Could you check a few things on this model? Use its own coordinates, in mm. Face numbers are marked on the shaded views. A direction names the side the tool comes from. Round coordinates to 2 decimals unless told otherwise and drop trailing zeros. Loops run counter-clockwise (first coordinate to the right, second up) from the corner with the lowest first, then second, coordinate; pieces in that order, holes last. Notation, with made-up numbers: (-21.75, -7) -> (31.25, -7) arc R30 ccw to (31.25, 32) -> close; hole circle Ø2 at (48.5, -31.5). An arc over 180 degrees is marked (long way). Write each question's results on one line, items separated by ' | '. Start each with the question number.
1) If I drill on probe 1 along Z at (x, y) = (-0.75, 39); probe 2 along Z at (x, y) = (-3.25, 6), over which ranges is the centre line in solid material (lowest first)?
2) Imagine slicing it at B-B, the plane x = -3.75. List the corners of the cut face in (y, z) for me.
3) Imagine slicing it at A-A, the plane y = 53.5. List the corners of the cut face in (x, z) for me.
4) For P1, Ø3, axis at y = 59, z = -4, coming from the -X side; P2, Ø2, axis at y = 58, z = -4, coming from the +X side, each with a flat end and sliding along its axis, tell me the tip position at first contact or that it passes through.
5) Which directions (+Z, -Z, +X, -X, +Y, -Y) give clear straight access to the entire face, cutting with the end or side of a thin tool? Please do the marked faces 1, 2 and 3.
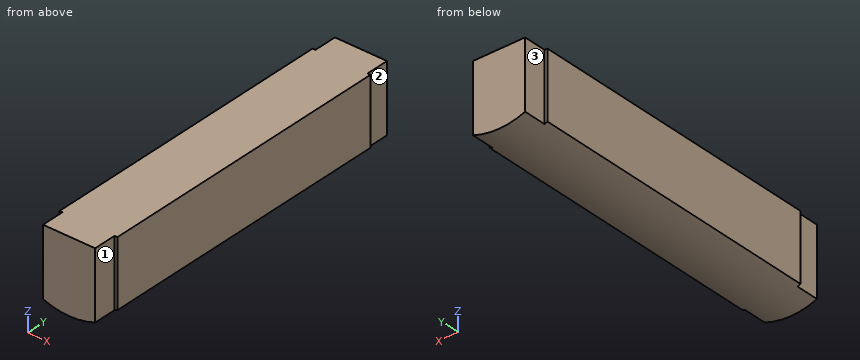
from build123d import *

# Parameters (mm, degrees)
BOSS_EXTRUDE1_DEPTH = 60
SKETCH3_W           = 0.5
SKETCH3_H           = 4
CUT_EXTRUDE1_DEPTH  = 20


with BuildPart() as part:
    # Sketch2 → Boss-Extrude1 (new body)
    with BuildSketch(Plane(origin=(0, 0, 0), x_dir=(1, 0, 0), z_dir=(0, 1, 0))):
        with BuildLine():
            Line((-5, 0), (5, 0))
            Line((5, 0), (5, 11.456439237))
            ThreePointArc((5, 11.456439237), (0, 12.5), (-5, 11.456439237))
            Line((-5, 11.456439237), (-5, 0))
        make_face()
    extrude(amount=BOSS_EXTRUDE1_DEPTH)

    # Sketch3 → Cut-Extrude1 (cut)
    with BuildSketch(Plane.XY):
        with Locations((-4.75, 2)):
            Rectangle(SKETCH3_W, SKETCH3_H)
        with Locations((4.75, 2)):
            Rectangle(SKETCH3_W, SKETCH3_H)
        with Locations((4.75, 58)):
            Rectangle(SKETCH3_W, SKETCH3_H)
        with Locations((-4.75, 58)):
            Rectangle(SKETCH3_W, SKETCH3_H)
    extrude(amount=-CUT_EXTRUDE1_DEPTH, mode=Mode.SUBTRACT)


solid = part.part
Checked values:
1) probe 1: -12.48 to 0 | probe 2: -12.07 to 0
2) outline: (0, -11.92) -> (60, -11.92) -> (60, 0) -> (0, 0) -> close
3) outline: (-5, -11.46) arc R12.5 ccw to (5, -11.46) -> (5, 0) -> (-5, 0) -> close
4) P1: x = -4.5 | P2: x = 4.5
5) face 1: +Z, -Z, +X, -Y | face 2: +Z, -Z, +X, +Y | face 3: +Z, -Z, -X, +Y
